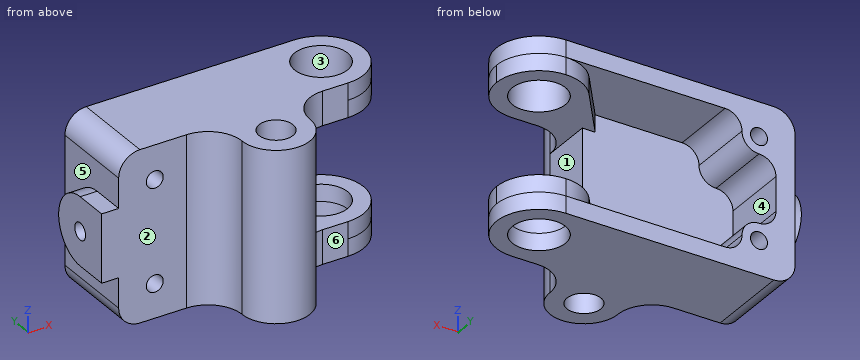
```python
from build123d import *

# Parameters (mm, degrees)
SKETCH1_R             = 8
SKETCH1_R_2           = 12.5
BOSS_EXTRUDE1_DEPTH   = 40
CUT_EXTRUDE1_DEPTH    = 32
SKETCH3_W             = 44
SKETCH3_H             = 64
CUT_EXTRUDE2_DEPTH    = 32
BOSS_EXTRUDE2_START   = 8
SKETCH4_R             = 12.5
BOSS_EXTRUDE2_DEPTH   = 8
F_8_0MM_DOWEL_HOLE1_D = 8
FILLET1_R             = 10
SKETCH6_R             = 4
BOSS_EXTRUDE3_DEPTH   = 8


with BuildPart() as part:
    # Sketch1 → Boss-Extrude1 (new, symmetric)
    with BuildSketch(Plane.XY):
        with BuildLine():
            Line((-64, 56), (-64, 16))
            Line((-64, 16), (-32, 16))
            ThreePointArc((-32, 16), (-20.686291501, 11.313708499), (-16, 0))
            ThreePointArc((-16, 0), (0, -16), (16, 0))
            ThreePointArc((16, 0), (20.686291501, 11.313708499), (32, 16))
            Line((32, 16), (44, 16))
            ThreePointArc((44, 16), (64, 36), (44, 56))
            Line((44, 56), (-64, 56))
        make_face()
        Circle(SKETCH1_R, mode=Mode.SUBTRACT)
        with Locations((44, 36)):
            Circle(SKETCH1_R_2, mode=Mode.SUBTRACT)
    extrude(amount=BOSS_EXTRUDE1_DEPTH, both=True)

    # Sketch2 → Cut-Extrude1 (cut)
    with BuildSketch(Plane(origin=(0, 56, 0), x_dir=(1, 0, 0), z_dir=(0, 1, 0))):
        with BuildLine():
            Line((64, 32), (-31, 32))
            ThreePointArc((-31, 32), (-36.656854249, 29.656854249), (-39, 24))
            ThreePointArc((-39, 24), (-41.343145751, 18.343145751), (-47, 16))
            ThreePointArc((-47, 16), (-52.656854249, 13.656854249), (-55, 8))
            Line((-55, 8), (-55, -8))
            ThreePointArc((-55, -8), (-52.656854249, -13.656854249), (-47, -16))
            ThreePointArc((-47, -16), (-41.343145751, -18.343145751), (-39, -24))
            ThreePointArc((-39, -24), (-36.656854249, -29.656854249), (-31, -32))
            Line((-31, -32), (64, -32))
            Line((64, -32), (64, 32))
        make_face()
    extrude(amount=-CUT_EXTRUDE1_DEPTH, mode=Mode.SUBTRACT)

    # Sketch3 → Cut-Extrude2 (cut)
    with BuildSketch(Plane(origin=(0, 24, 0), x_dir=(1, 0, 0), z_dir=(0, 1, 0))):
        with Locations((38, 0)):
            Rectangle(SKETCH3_W, SKETCH3_H)
    extrude(amount=-CUT_EXTRUDE2_DEPTH, mode=Mode.SUBTRACT)

    # Sketch4 → Boss-Extrude2 (add)
    # profile 1 of 2: a face of its own
    with BuildSketch(Plane.XY.offset(-32).offset(BOSS_EXTRUDE2_START)):
        with BuildLine():
            ThreePointArc((44, 56), (35.076043738, 53.898687232), (28.027289799, 48.036300463))
            ThreePointArc((28.027289799, 48.036300463), (26.101312768, 27.076043738), (44, 16))
            ThreePointArc((44, 16), (58.142135624, 21.857864376), (64, 36))
            ThreePointArc((64, 36), (58.142135624, 50.142135624), (44, 56))
        make_face()
        with Locations((44, 36)):
            Circle(SKETCH4_R, mode=Mode.SUBTRACT)
    # profile 2 of 2: a face of its own
    with BuildSketch(Plane.XY.offset(-32).offset(BOSS_EXTRUDE2_START)):
        with BuildLine():
            ThreePointArc((44, 16), (26.101312768, 27.076043738), (28.027289799, 48.036300463))
            Line((28.027289799, 48.036300463), (9.914638236, 24))
            Line((9.914638236, 24), (16, 24))
            Line((16, 24), (16, 0))
            ThreePointArc((16, 0), (20.686291501, 11.313708499), (32, 16))
            Line((32, 16), (44, 16))
        make_face()
    boss_extrude2 = extrude(amount=-BOSS_EXTRUDE2_DEPTH)

    # Mirror1: Boss-Extrude2 across plane
    add(boss_extrude2.mirror(Plane.XY))

    # Ø8.0mm Dowel Hole1 (through all)
    with Locations(Plane(origin=(-47, 56, -24), x_dir=(1, 0, 0), z_dir=(0, 1, 0))):
        with Locations((0, 0), (0, -48)):
            Hole(F_8_0MM_DOWEL_HOLE1_D / 2)

    # Fillet1
    fillet1_edges = [part.edges().sort_by_distance(p)[0] for p in [
        (-64, 36, -40),
        (-64, 36, 40),
    ]]
    fillet(fillet1_edges, radius=FILLET1_R)

    # Sketch6 → Boss-Extrude3 (add)
    with BuildSketch(Plane.ZY.offset(64)):
        with BuildLine():
            Line((-16, 16), (-16, 32))
            ThreePointArc((-16, 32), (0, 48), (16, 32))
            Line((16, 32), (16, 16))
            Line((16, 16), (-16, 16))
        make_face()
        with Locations((0, 32)):
            Circle(SKETCH6_R, mode=Mode.SUBTRACT)
    extrude(amount=BOSS_EXTRUDE3_DEPTH)


solid = part.part
```
The listing builds one solid part. Answer for the finished solid, in the listing's coordinates (mm). Face numbers are marked on the shaded views. A direction names the side the tool comes from. Give positions to 0.01 mm unless a question says otherwise; leave off trailing zeros. Write each loop counter-clockwise with the first axis right and the second up, starting at its lowest first coordinate (ties: lowest second). Pieces come first, ordered by that corner, then holes. Notation, with made-up numbers: (77, -32) -> (114, -32) arc R24 cw to (114, -11) -> close; hole circle Ø7 at (-18, 4). An arc over 180 degrees is marked (long way). Write item = value, one per line. Start each with the question number.
1) The part is cut by section B-B, the plane x = 0. Determine the outline of the cut face in (y, z).
2) The part is cut by section C-C, the plane x = 52.5. Determine the outline of the cut face in (y, z), and give its area (3 significant figures).
3) Determine the mould class of the marked faces 1, 2 and 3 for opening direction Y: +Y half, -Y half, draft (parallel to the pull), parting line (faces both ways), or undercut.
4) Straight lines are drawn through the part: line 1 along Z through (x, y) = (-47, 35); line 2 along X through (y, z) = (-0.5, 37); line 3 along Y through (x, z) = (-67, 0). For each, find the intervals that lie inside material, in ascending order.
5) The part is cut by section D-D, the plane x = 18. Determine the outline of the cut face in (y, z).
6) The part is cut by section A-A, the plane z = 0. Determine the outline of the cut face in (x, y), and give its area (3 significant figures).
7) Each of these flat-tipped pins is pushed along its axis until it touches: pin 1 (8 mm diameter, centred on y = 45, z = -1.5, fed in from +X); pin 2 (4 mm diameter, centred on y = 34, z = 0.5, fed in from -X); pin 3 (3.5 mm diameter, centred on x = 40.5, z = 29.5, fed in from -Y); pin 4 (4 mm diameter, centred on x = -69.5, y = 22.5, fed in from +Z). Where does it stop, or does it pass through?
8) Which of the six approach directions +Z, -Z, +X, -X, +Y, -Y give full straight-line access (tool end or side, diameter ignored) to the marked faces 4, 5 and 6?
Solutions:
q1.outline = (-16, -40) -> (-8, -40) -> (-8, 40) -> (-16, 40) -> close; (8, -40) -> (56, -40) -> (56, -32) -> (24, -32) -> (24, 32) -> (56, 32) -> (56, 40) -> (8, 40) -> close
q2.outline = (17.9, -40) -> (26.83, -40) -> (26.83, -24) -> (17.9, -24) -> close; (17.9, 24) -> (26.83, 24) -> (26.83, 40) -> (17.9, 40) -> close; (45.17, -40) -> (54.1, -40) -> (54.1, -24) -> (45.17, -24) -> close; (45.17, 24) -> (54.1, 24) -> (54.1, 40) -> (45.17, 40) -> close
q2.area = 572 mm²
q3.face_1 = draft
q3.face_2 = -Y half
q3.face_3 = undercut
q4.line_1 = -40 to -28, -20 to -16, 16 to 20, 28 to 40
q4.line_2 = -15.99 to -7.98, 7.98 to 15.99
q4.line_3 = 16 to 28, 36 to 48
q5.outline = (7.75, -40) -> (56, -40) -> (56, -32) -> (34.73, -32) -> (34.73, -24) -> (7.75, -24) -> close; (7.75, 24) -> (34.73, 24) -> (34.73, 32) -> (56, 32) -> (56, 40) -> (7.75, 40) -> close
q6.outline = (-72, 16) -> (-32, 16) arc R16 cw to (-16, 0) arc R16 ccw to (16, 0) -> (16, 24) -> (-55, 24) -> (-55, 56) -> (-64, 56) -> (-64, 48) -> (-72, 48) -> (-72, 36) -> (-64, 36) -> (-64, 28) -> (-72, 28) -> close; hole circle Ø16 at (0, 0)
q6.area = 1,890 mm²
q7.pin_1 = -55
q7.pin_2 = -72
q7.pin_3 = 16
q7.pin_4 = 16
q8.face_4 = +X, +Y
q8.face_5 = -X, +Y
q8.face_6 = +Z, -Z, +X, -Y
